Design review of the part built by this model. Coordinates are the model's own, in mm. A direction names the side the tool comes from. Coordinates: 2 decimals unless noted, no trailing zeros. Loops run counter-clockwise (first coordinate to the right, second up) from the corner with the lowest first, then second, coordinate; pieces in that order, holes last. Notation, with made-up numbers: (13.25, 0.25) -> (25.25, 0.25) arc R18 cw to (25.25, 13.25) -> close; hole circle Ø11 at (41, 77). An arc over 180 degrees is marked (long way). Use one line per item in the form item = value. Start each with the question number.
1. Consider section D-D (z = 0.7). State the section outline as (x, y) points.
2. Wall thickness on line 1 (Y direction, x = 0, z = 0.4); line 2 (X direction, y = -27, z = 1.8); line 3 (Y direction, x = -1, z = 0.8): over which ranges is each line inside the solid? List them lowest first. Write a range as from..to.
3. For pin 1 (2 mm diameter, centred on x = -26, z = -1.5, fed in from +Y), flat-tipped, find the tip position at first contact; note if it passes through.
4. Machinability: for faces 1 (the face through (26, -13.437, 0)), 2 (the face through (1, -8, -2.388)), 3 (the face through (-11.963, 13, 0)), which of the approach directions +Z, -Z, +X, -X, +Y, -Y give a long, thin tool a straight path to every point of the face, cutting with its end or side? Answer none if there is none.
5. Consider section B-B (x = 25.4). State the section outline as (y, z) points.
6. Consider section A-A (x = 0). State the section outline as (y, z) points, then the cut area to 3 significant figures.
7. The part is to be moulded in two halves that separate along Y. For faces 4 (the face through (-23.89, -28.66, 0.03)), 5 (the face through (-26, -13.437, 0)), 6 (the face through (38.1, -26, 0)), 7 (the face through (1, -38.1, 0)), say which applies: released by +Y, released by -Y, zero draft, split by the parting line, or undercut.
8. Consider section C-C (y = 2). State the section outline as (x, z) points, then the cut area to 3 significant figures.
from build123d import *

# Parameters (mm, degrees)
BOSS_EXTRUDE1_DEPTH      = 2.3876
BOSS_EXTRUDE1_DEPTH_BACK = 2.3876
SKETCH4_R                = 3.2639
CUT_EXTRUDE1_DEPTH       = 55.092721646


with BuildPart() as part:
    # Sketch3 → Boss-Extrude1 (new, two sides: drawn at the far end of the back side and taken through both)
    with BuildSketch(Plane.XY.offset(-BOSS_EXTRUDE1_DEPTH_BACK)):
        with BuildLine():
            Line((38.1, -38.1), (-38.1, -38.1))
            Line((-38.1, -38.1), (-38.1, -13.4366))
            Line((-38.1, -13.4366), (-14.351, -13.4366))
            ThreePointArc((-14.351, -13.4366), (-12.662711849, -12.737288151), (-11.9634, -11.049))
            Line((-11.9634, -11.049), (-11.9634, 38.1))
            Line((-11.9634, 38.1), (11.9634, 38.1))
            Line((11.9634, 38.1), (11.9634, -11.049))
            ThreePointArc((11.9634, -11.049), (12.662711849, -12.737288151), (14.351, -13.4366))
            Line((14.351, -13.4366), (38.1, -13.4366))
            Line((38.1, -13.4366), (38.1, -38.1))
        make_face()
    extrude(amount=BOSS_EXTRUDE1_DEPTH + BOSS_EXTRUDE1_DEPTH_BACK)

    # Sketch4 → Cut-Extrude1 (cut, through all)
    with BuildSketch(Plane.XY.offset(2.3876)):
        with Locations((25.4, -25.7683)):
            Circle(SKETCH4_R)
        with Locations((0, -25.7683)):
            Circle(SKETCH4_R)
        with Locations((-25.4, -25.7683)):
            Circle(SKETCH4_R)
        with Locations((0, -0.3683)):
            Circle(SKETCH4_R)
        with Locations(Location((0, 25.0317, 0), (0, 0, 180))):
            Circle(SKETCH4_R)
    extrude(amount=-CUT_EXTRUDE1_DEPTH, mode=Mode.SUBTRACT)


solid = part.part
Geometry check:
q1.outline = (-38.1, -38.1) -> (38.1, -38.1) -> (38.1, -13.44) -> (14.35, -13.44) arc R2.39 cw to (11.96, -11.05) -> (11.96, 38.1) -> (-11.96, 38.1) -> (-11.96, -11.05) arc R2.39 cw to (-14.35, -13.44) -> (-38.1, -13.44) -> close; hole circle Ø6.53 at (-25.4, -25.77); hole circle Ø6.53 at (0, -25.77); hole circle Ø6.53 at (0, -0.37); hole circle Ø6.53 at (0, 25.03); hole circle Ø6.53 at (25.4, -25.77)
q2.line_1 = -38.1..-29.03, -22.5..-3.63, 2.9..21.77, 28.3..38.1
q2.line_2 = -38.1..-28.42, -22.38..-3.02, 3.02..22.38, 28.42..38.1
q2.line_3 = -38.1..-28.88, -22.66..-3.48, 2.74..21.92, 28.14..38.1
q3.pin_1 = -13.44
q4.face_1 = +Z, -Z, +X, +Y
q4.face_2 = -Z, +X, -X, +Y, -Y
q4.face_3 = +Z, -Z, -X, +Y
q5.outline = (-38.1, -2.39) -> (-29.03, -2.39) -> (-29.03, 2.39) -> (-38.1, 2.39) -> close; (-22.5, -2.39) -> (-13.44, -2.39) -> (-13.44, 2.39) -> (-22.5, 2.39) -> close
q6.outline = (-38.1, -2.39) -> (-29.03, -2.39) -> (-29.03, 2.39) -> (-38.1, 2.39) -> close; (-22.5, -2.39) -> (-3.63, -2.39) -> (-3.63, 2.39) -> (-22.5, 2.39) -> close; (2.9, -2.39) -> (21.77, -2.39) -> (21.77, 2.39) -> (2.9, 2.39) -> close; (28.3, -2.39) -> (38.1, -2.39) -> (38.1, 2.39) -> (28.3, 2.39) -> close
q6.area = 270 mm²
q7.face_4 = undercut
q7.face_5 = released by +Y
q7.face_6 = zero draft
q7.face_7 = released by -Y
q8.outline = (-11.96, -2.39) -> (-2.25, -2.39) -> (-2.25, 2.39) -> (-11.96, 2.39) -> close; (2.25, -2.39) -> (11.96, -2.39) -> (11.96, 2.39) -> (2.25, 2.39) -> close
q8.area = 92.8 mm²
